```python
from build123d import *

# Parameters (mm, degrees)
BOSS_EXTRUDE1_DEPTH = 9
CHAMFER1_SIZE       = 1
SKETCH2_R           = 2
CUT_EXTRUDE1_DEPTH  = 25
CUT_EXTRUDE2_START  = -7
SKETCH2_3_R         = 3
SKETCH2_3_R_2       = 2
CUT_EXTRUDE2_DEPTH  = 15
CUT_EXTRUDE3_START  = 24
SKETCH2_4_R         = 3
SKETCH2_4_R_2       = 2
CUT_EXTRUDE3_DEPTH  = 17


with BuildPart() as part:
    # Sketch1 → Boss-Extrude1 (new body)
    with BuildSketch(Plane(origin=(0, 0, 0), x_dir=(1, 0, 0), z_dir=(0, 1, 0))):
        with BuildLine():
            Line((-0.75, 21), (-0.75, 17.483921185))
            ThreePointArc((-0.75, 17.483921185), (-17.5, 0), (-0.75, -17.483921185))
            Line((-0.75, -17.483921185), (-0.75, -26.489384666))
            ThreePointArc((-0.75, -26.489384666), (0, 26.5), (0.75, -26.489384666))
            Line((0.75, -26.489384666), (0.75, -17.483921185))
            ThreePointArc((0.75, -17.483921185), (17.5, 0), (0.75, 17.483921185))
            Line((0.75, 17.483921185), (0.75, 21))
            Line((0.75, 21), (-0.75, 21))
        make_face()
    extrude(amount=BOSS_EXTRUDE1_DEPTH)

    # Chamfer1
    chamfer1_edges = [part.edges().sort_by_distance(p)[0] for p in [
        (17.5, 0, 0),
        (17.5, 9, 0),
        (0, 9, -26.5),
        (-17.5, 9, 0),
        (-17.5, 0, 0),
        (0, 0, -26.5),
    ]]
    chamfer(chamfer1_edges, length=CHAMFER1_SIZE)

    # Sketch2 → Cut-Extrude1 (cut, symmetric)
    with BuildSketch(Plane(origin=(0, 0, 0), x_dir=(0, 0, -1), z_dir=(1, 0, 0))):
        with Locations((-21.983921185, 4.5)):
            Circle(SKETCH2_R)
    extrude(amount=CUT_EXTRUDE1_DEPTH, both=True, mode=Mode.SUBTRACT)

    # Sketch2<3> → Cut-Extrude2 (cut)
    with BuildSketch(Plane(origin=(0, 0, 0), x_dir=(0, 0, -1), z_dir=(1, 0, 0)).offset(CUT_EXTRUDE2_START)):
        with Locations((-21.983921185, 4.5)):
            Circle(SKETCH2_3_R)
        with Locations((-21.983921185, 4.5)):
            Circle(SKETCH2_3_R_2, mode=Mode.SUBTRACT)
    extrude(amount=-CUT_EXTRUDE2_DEPTH, mode=Mode.SUBTRACT)

    # Sketch2<4> → Cut-Extrude3 (cut)
    with BuildSketch(Plane(origin=(0, 0, 0), x_dir=(0, 0, -1), z_dir=(1, 0, 0)).offset(CUT_EXTRUDE3_START)):
        with Locations((-21.983921185, 4.5)):
            Circle(SKETCH2_4_R)
        with Locations((-21.983921185, 4.5)):
            Circle(SKETCH2_4_R_2, mode=Mode.SUBTRACT)
    extrude(amount=-CUT_EXTRUDE3_DEPTH, mode=Mode.SUBTRACT)


solid = part.part
```
Build history of the part. All positions in model axes, mm. A direction names the side the tool comes from. Round coordinates to 2 decimals unless told otherwise and drop trailing zeros. Order: outer loops, then holes, each group sorted by start corner. A loop starts at its lowest first (then second) coordinate and runs counter-clockwise, first axis right, second up. Notation, with made-up numbers: (19.5, -39) -> (58.5, -39) arc R19 cw to (58.5, -12) -> close; hole circle Ø6 at (28, 54.5). An arc over 180 degrees is marked (long way). Answer in a Markdown table with one row per item.
1) Band-saw the part on A-A on z = 0. Give the cut face in (x, y), and give its area (3 significant figures).
Values:
| item | result |
|---|---|
| outline | (-26.5, 1) -> (-25.5, 0) -> (-18.5, 0) -> (-17.5, 1) -> (-17.5, 8) -> (-18.5, 9) -> (-25.5, 9) -> (-26.5, 8) -> close; (17.5, 1) -> (18.5, 0) -> (25.5, 0) -> (26.5, 1) -> (26.5, 8) -> (25.5, 9) -> (18.5, 9) -> (17.5, 8) -> close |
| area | 158 mm2 |
2) Band-saw the part on D-D on x = 0. Give the cut face in (y, z), and give its area (3 significant figures).
Values:
| item | result |
|---|---|
| outline | (0, -25.5) -> (1, -26.5) -> (8, -26.5) -> (9, -25.5) -> (9, -21) -> (0, -21) -> close |
| area | 48.5 mm2 |
3) Mould opens along Y. For faces 1 (the flat face through (-7, 7, 22)), 2 (the flat face through (0.75, 4, -19)), 3 (the flat face through (13.3, 9, 13.1)) say: released by +Y, released by -Y, zero draft, split by the parting line, or undercut.
Values:
| item | result |
|---|---|
| face 1 | undercut |
| face 2 | zero draft |
| face 3 | released by +Y |
4) Wall check: L1, parallel to X at y = 1, z = 19; L2, parallel to Z at x = 5.5, y = 4.25; L3, parallel to X at y = 1, z = 0.5. Give the ranges that are in metal, low to high.
Values:
| item | result |
|---|---|
| L1 | -18.47 to -0.75, 0.75 to 18.47 |
| L2 | -25.92 to -16.61, 16.61 to 20, 23.97 to 25.92 |
| L3 | -26.5 to -17.49, 17.49 to 26.5 |
5) Pin check, flat tips, straight feed: P1, Ø2, axis at y = 6, z = 14.5, coming from the +X side; P2, Ø1.5, axis at x = 13, z = -9.5, coming from the -Y side; P3, Ø3, axis at y = 3, z = -20, coming from the +X side; P4, Ø3, axis at x = 16.5, y = 1.5, coming from the -Z side. Stop position of each tip, or through.
Values:
| item | result |
|---|---|
| P1 | x = 22.8 |
| P2 | through |
| P3 | x = 18.97 |
| P4 | z = -21.85 |
6) Band-saw the part on B-B on y = 4.5. Give the cut face in (x, z).
Values:
| item | result |
|---|---|
| outline | (-18.49, 18.98) arc R26.5 ccw (long way) to (18.49, 18.98) -> (7, 18.98) -> (7, 19.98) -> (0.75, 19.98) -> (0.75, 17.48) arc R17.5 cw to (0.75, -17.48) -> (0.75, -21) -> (-0.75, -21) -> (-0.75, -17.48) arc R17.5 cw to (-0.75, 17.48) -> (-0.75, 19.98) -> (-7, 19.98) -> (-7, 18.98) -> close; (-8.83, 24.98) -> (-7, 24.98) -> (-7, 23.98) -> (-0.75, 23.98) -> (-0.75, 26.49) arc R26.5 ccw to start; (0.75, 23.98) -> (7, 23.98) -> (7, 24.98) -> (8.83, 24.98) arc R26.5 ccw to (0.75, 26.49) -> close |
7) Which spindle directions (+Z, -Z, +X, -X, +Y, -Y) get a long thin tool onto all of the face, cutting with end or side? Do faces 4 (the conical face through (17.67, 0.826, 0.379)), 5 (the flat face through (7, 7, 22)), 6 (the flat face through (0, 4, -21)), 7 (the cylindrical face through (-11.388, 5.401, 19.122)). Say none if no direction does.
Values:
| item | result |
|---|---|
| face 4 | -Y |
| face 5 | +X |
| face 6 | +Z, +Y, -Y |
| face 7 | -X |
8) Band-saw the part on C-C on x = 6. Give the number of separate pieces and of enclosed holes in the cut face, and give its area (3 significant figures).
Values:
| item | result |
|---|---|
| separate pieces | 2 |
| enclosed holes | 1 |
| area | 152 mm2 |
